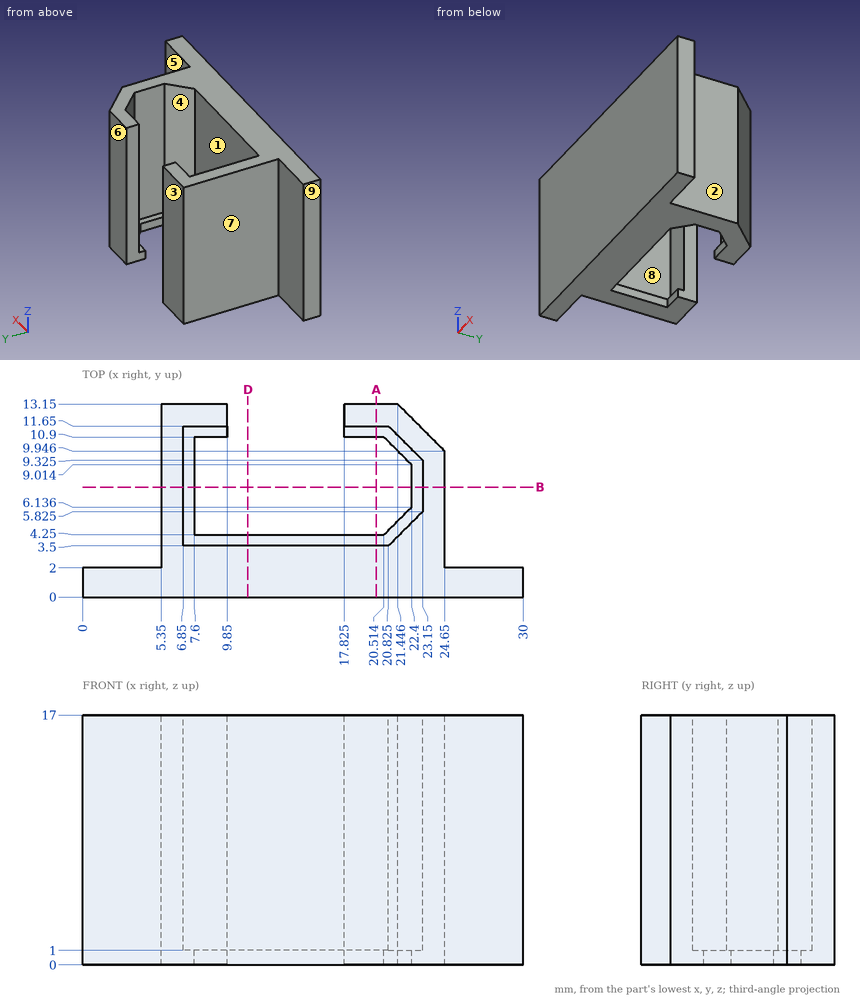
Study the drawing (mm; zero at the part's minimum x, y, z) and answer. A direction names the side the tool comes from. Give positions to 0.01 mm unless a question says otherwise; leave off trailing zeros. Write each loop counter-clockwise with the first axis right and the second up, starting at its lowest first coordinate (ties: lowest second). Pieces come first, ordered by that corner, then holes.
Item 1: Find the intervals of material crossed by line 1 along Y through (x, z) = (9.75, 10); line 2 along Z through (x, y) = (8.25, 11); line 3 along Y through (x, z) = (16.25, 14.25), in increasing order.
Item 2: Determine the mould class of the marked faces 1, 2, 3 and 4 for opening direction X: released by +X, released by -X, zero draft, split by the parting line, or undercut.
Item 3: Section A-A, the plane x = 20 is taken. Write down the section's boundary in (y, z).
Item 4: Which of the six approach directions +Z, -Z, +X, -X, +Y, -Y give full straight-line access (tool end or side, diameter ignored) to the marked faces 5, 6, 7, 8 and 9?
Item 5: Section B-B, the plane y = 7.5 is taken. Write down the section's boundary in (x, z).
Item 6: Section D-D, the plane x = 11.25 is taken. Write down the section's boundary in (y, z).
Item 7: Flat-ended cylindrical pins translate along their axes: P1, Ø0.8, axis at y = 8, z = 0.5, coming from the -X side; P2, Ø1, axis at x = 21, y = 10.5, coming from the +Z side; P3, Ø5, axis at y = 6, z = 12.5, coming from the +X side. Find the tip coordinate at first contact, or state that the pin passes through.
Completed:
1. line 1: y = 0 to 3.5, 11.65 to 13.15
1. line 2: z = 0 to 1
1. line 3: y = 0 to 3.5
2. face 1: undercut
2. face 2: released by +X
2. face 3: zero draft
2. face 4: undercut
3. outline: (0, 0) - (4.25, 0) - (4.25, 1) - (3.5, 1) - (3.5, 17) - (0, 17) - close; (10.9, 0) - (13.15, 0) - (13.15, 17) - (11.65, 17) - (11.65, 1) - (10.9, 1) - close
4. face 5: +Z, -Z, +X, +Y
4. face 6: +Z, -Z, +X, -X, +Y
4. face 7: +Z, -Z, -X, +Y
4. face 8: +Z
4. face 9: +Z, -Z, -X, +Y, -Y
5. outline: (5.35, 0) - (7.6, 0) - (7.6, 1) - (6.85, 1) - (6.85, 17) - (5.35, 17) - close; (22.4, 0) - (24.65, 0) - (24.65, 17) - (23.15, 17) - (23.15, 1) - (22.4, 1) - close
6. outline: (0, 0) - (4.25, 0) - (4.25, 1) - (3.5, 1) - (3.5, 17) - (0, 17) - close
7. P1: stops at x = 5.35
7. P2: stops at z = 1
7. P3: stops at x = 24.65
